CAD build for the part. Positions are in the model's coordinates, mm. A direction names the side the tool comes from. Give positions to 0.01 mm unless a question says otherwise; leave off trailing zeros. Loops run counter-clockwise (first coordinate to the right, second up) from the corner with the lowest first, then second, coordinate; pieces in that order, holes last.
```python
from build123d import *

# Parameters (mm, degrees)
SKETCH1_W           = 115
SKETCH1_H           = 30
BOSS_EXTRUDE1_DEPTH = 5
SKETCH2_W           = 5
SKETCH2_H           = 30
BOSS_EXTRUDE2_DEPTH = 30
SKETCH3_R           = 8.75
BOSS_EXTRUDE3_DEPTH = 5
SKETCH4_R           = 1.95
BOSS_EXTRUDE4_DEPTH = 1.9
CIRPATTERN1_COUNT   = 4
SKETCH5_W           = 115
SKETCH5_H           = 35
BOSS_EXTRUDE5_DEPTH = 5
SKETCH6_R           = 1.55
CUT_EXTRUDE2_DEPTH  = 124.895116934
SKETCH7_R           = 1.35
CUT_EXTRUDE3_DEPTH  = 10
SKETCH8_R           = 3.25
CUT_EXTRUDE4_DEPTH  = 3
SKETCH9_W           = 7
SKETCH9_H           = 20
CUT_EXTRUDE5_DEPTH  = 5
SKETCH10_R          = 4.5
BOSS_EXTRUDE6_DEPTH = 10


with BuildPart() as part:
    # Sketch1 → Boss-Extrude1 (new body)
    with BuildSketch(Plane(origin=(0, 0, 0), x_dir=(1, 0, 0), z_dir=(0, 1, 0))):
        with Locations((57.5, -15)):
            Rectangle(SKETCH1_W, SKETCH1_H)
    extrude(amount=BOSS_EXTRUDE1_DEPTH)

    # Sketch2 → Boss-Extrude2 (add)
    with BuildSketch(Plane(origin=(0, 5, 0), x_dir=(1, 0, 0), z_dir=(0, 1, 0))):
        with Locations((2.5, -15)):
            Rectangle(SKETCH2_W, SKETCH2_H)
        with Locations((112.5, -15)):
            Rectangle(SKETCH2_W, SKETCH2_H)
    extrude(amount=BOSS_EXTRUDE2_DEPTH)

    # Sketch3 → Boss-Extrude3 (add)
    with BuildSketch(Plane.ZY):
        with Locations((15, 23)):
            Circle(SKETCH3_R)
    extrude(amount=BOSS_EXTRUDE3_DEPTH)

    # Sketch4 → Boss-Extrude4 (add)
    with BuildSketch(Plane.ZY.offset(5)):
        with Locations(Location((15, 29, 0), (0, 0, 180))):
            Circle(SKETCH4_R)
    boss_extrude4 = extrude(amount=BOSS_EXTRUDE4_DEPTH)

    # CirPattern1: Boss-Extrude4 ×4 about axis
    cirpattern1_axis = Axis((0, 23, 15), (1, 0, 0))
    for i in range(1, CIRPATTERN1_COUNT):
        add(boss_extrude4.rotate(cirpattern1_axis, i * 360 / CIRPATTERN1_COUNT))

    # Sketch5 → Boss-Extrude5 (add)
    with BuildSketch(Plane.XY.offset(30)):
        with Locations((57.5, 17.5)):
            Rectangle(SKETCH5_W, SKETCH5_H)
    extrude(amount=BOSS_EXTRUDE5_DEPTH)

    # Sketch6 → Cut-Extrude2 (cut, through all)
    with BuildSketch(Plane(origin=(0, 0, 30), x_dir=(-1, 0, 0), z_dir=(0, 0, -1))):
        with Locations((-80, 17.5)):
            Circle(SKETCH6_R)
        with Locations((-35, 17.5)):
            Circle(SKETCH6_R)
    extrude(amount=-CUT_EXTRUDE2_DEPTH, mode=Mode.SUBTRACT)

    # Sketch7 → Cut-Extrude3 (cut)
    with BuildSketch(Plane.ZY.offset(5)):
        with Locations((15, 23)):
            Circle(SKETCH7_R)
    extrude(amount=-CUT_EXTRUDE3_DEPTH, mode=Mode.SUBTRACT)

    # Sketch8 → Cut-Extrude4 (cut)
    with BuildSketch(Plane(origin=(5, 0, 0), x_dir=(0, 0, -1), z_dir=(1, 0, 0))):
        with Locations((-15, 23)):
            Circle(SKETCH8_R)
    extrude(amount=-CUT_EXTRUDE4_DEPTH, mode=Mode.SUBTRACT)

    # Sketch9 → Cut-Extrude5 (cut)
    with BuildSketch(Plane(origin=(115, 0, 0), x_dir=(0, 0, -1), z_dir=(1, 0, 0))):
        with Locations((-26.5, 15)):
            Rectangle(SKETCH9_W, SKETCH9_H)
    extrude(amount=-CUT_EXTRUDE5_DEPTH, mode=Mode.SUBTRACT)

    # Sketch10 → Boss-Extrude6 (add)
    with BuildSketch(Plane(origin=(115, 0, 0), x_dir=(0, 0, -1), z_dir=(1, 0, 0))):
        with Locations(Location((-15, 23, 0), (0, 0, 180))):
            Circle(SKETCH10_R)
    extrude(amount=BOSS_EXTRUDE6_DEPTH)


solid = part.part
```
1. Pull direction Y, two halves, no side cores. Call faces 1 (the face through (-5.937, 17.086, 13.052)), 2 (the face through (57, 0, 17)), 3 (the face through (-2.46, 28.91, 8.55)), 4 (the face through (115, 17, 17)): released by +Y, released by -Y, zero draft, split by the parting line, or undercut.
Responses:
face 1: undercut
face 2: released by -Y
face 3: split by the parting line
face 4: zero draft
2. Drop flat-ended pins along their axis: pin 1 (4 mm diameter, centred on y = 23, z = 15, fed in from -X); pin 2 (5.5 mm diameter, centred on x = 111.5, z = 26.5, fed in from -Y); pin 3 (1.6 mm diameter, centred on y = 23, z = 15, fed in from -X); pin 4 (8 mm diameter, centred on y = 15, z = 22.5, fed in from +X). Give the stop position or say it passes through.
Responses:
pin 1: stops at x = -5
pin 2: stops at y = 0
pin 3: stops at x = 110
pin 4: stops at x = 115
3. Probe line 1 along Y through (x, z) = (80, 33); line 2 along Y through (x, z) = (3.45, 15); line 3 along X through (y, z) = (11, 12). List the from-to ranges inside material, lowest first.
Responses:
line 1: y = 0 to 15.95, 19.05 to 35
line 2: y = 0 to 19.75, 26.25 to 35
line 3: x = 0 to 5, 110 to 115
4. Saw through at D-D, the plane y = 23. Count the separate pieces of the cut face and the enclosed holes in it, and give its area (3 significant figures).
Responses:
separate pieces: 3
enclosed holes: 0
area: 994 mm2
5. Saw through at C-C, the plane y = 9. List the corners of the cut face in (x, z).
Responses:
outline: (0, 0) - (5, 0) - (5, 30) - (115, 30) - (115, 35) - (0, 35) - close; (110, 0) - (115, 0) - (115, 23) - (110, 23) - close
6. Saw through at A-A, the plane x = 80. List the corners of the cut face in (y, z), and give its area (4 significant figures).
Responses:
outline: (0, 0) - (5, 0) - (5, 30) - (15.95, 30) - (15.95, 35) - (0, 35) - close; (19.05, 30) - (35, 30) - (35, 35) - (19.05, 35) - close
area: 309.5 mm2
7. Tool access for faces 5 (the face through (119.93, 18.54, 14.41)), 6 (the face through (57, 18, 35)), 7 (the face through (3.521, 21.022, 17.579)), 8 (the face through (-5, 21, 15)): list every direction of +Z, -Z, +X, -X, +Y, -Y with a clear straight run to the whole face (end or side of a thin tool).
Responses:
face 5: +X
face 6: +Z, +X, -X, +Y, -Y
face 7: none
face 8: -X
